```python
from build123d import *

# Parameters (mm, degrees)
CASING_SKETCH_W        = 150
CASING_SKETCH_H        = 200
CASING_DEPTH           = 100
SHELL1_T               = -2
COMPARTMENTS_OUTLINE_W = 146
COMPARTMENTS_OUTLINE_H = 2
COMPARTMENTS_DEPTH     = 100
SKETCH4_W              = 51
SKETCH4_H              = 60
SKETCH4_W_2            = 35
SKETCH4_H_2            = 40
SKETCH4_W_3            = 30
SKETCH4_H_3            = 100
SKETCH4_W_4            = 70
SKETCH4_H_4            = 30
MEDICINES_DEPTH        = 75
SKETCH6_R              = 17.5
SKETCH6_R_2            = 5
BANDAGE_DEPTH          = 75
SKETCH7_R              = 7.5
VIALS_DEPTH            = 25
SKETCH9_W              = 150
SKETCH9_H              = 200
BOSS_EXTRUDE1_DEPTH    = 2
CUT_EXTRUDE1_DEPTH     = 2


# Read off the part's stored shape, not the designer's step: Compartments
with BuildPart() as part:
    # Casing Sketch → Casing (new body)
    with BuildSketch(Plane(origin=(0, 0, 0), x_dir=(1, 0, 0), z_dir=(0, 1, 0))):
        Rectangle(CASING_SKETCH_W, CASING_SKETCH_H)
    extrude(amount=CASING_DEPTH)

    # Shell1
    shell1_openings = [part.faces().sort_by_distance(p)[0] for p in [
        (0, 100, 0),
    ]]
    offset(amount=SHELL1_T, openings=shell1_openings, kind=Kind.INTERSECTION)

    # Compartments outline → Compartments (add)
    with BuildSketch(Plane(origin=(0, 2, 0), x_dir=(1, 0, 0), z_dir=(0, 1, 0))):
        Polygon((-2, 2), (-73, 2), (-73, 0), (0, 0), (0, 98), (-2, 98), align=None)
        with Locations((0, -51)):
            Rectangle(COMPARTMENTS_OUTLINE_W, COMPARTMENTS_OUTLINE_H)
    extrude(amount=COMPARTMENTS_DEPTH)

    # Sketch4 → Medicines (add)
    with BuildSketch(Plane(origin=(0, 2, 0), x_dir=(1, 0, 0), z_dir=(0, 1, 0))):
        with Locations((-37.5, 32)):
            Rectangle(SKETCH4_W, SKETCH4_H)
        with Locations((15.5, -30)):
            Rectangle(SKETCH4_W_2, SKETCH4_H_2)
        with Locations((53, 0)):
            Rectangle(SKETCH4_W_3, SKETCH4_H_3)
        with Locations((-28, -83)):
            Rectangle(SKETCH4_W_4, SKETCH4_H_4)
    extrude(amount=MEDICINES_DEPTH)

    # Sketch6 → Bandage (add)
    with BuildSketch(Plane(origin=(0, 2, 0), x_dir=(1, 0, 0), z_dir=(0, 1, 0))):
        with Locations(Location((43.231606139, -78.51417502, 0), (0, 0, 270))):
            Circle(SKETCH6_R)
        with Locations(Location((43.231606139, -78.51417502, 0), (0, 0, 270))):
            Circle(SKETCH6_R_2, mode=Mode.SUBTRACT)
    extrude(amount=BANDAGE_DEPTH)

    # Sketch7 → Vials (add)
    with BuildSketch(Plane(origin=(0, 0, 50), x_dir=(-1, 0, 0), z_dir=(0, 0, -1))):
        with Locations((61.244974069, 52)):
            Circle(SKETCH7_R)
        with Locations((37.16355204, 52)):
            Circle(SKETCH7_R)
        with Locations((14.684505224, 52)):
            Circle(SKETCH7_R)
    extrude(amount=VIALS_DEPTH)

    # Sketch9 → Boss-Extrude1 (add)
    with BuildSketch(Plane(origin=(0, 100, 0), x_dir=(1, 0, 0), z_dir=(0, 1, 0))):
        Rectangle(SKETCH9_W, SKETCH9_H)
    extrude(amount=BOSS_EXTRUDE1_DEPTH)

    # Sketch10 → Cut-Extrude1 (cut)
    with BuildSketch(Plane(origin=(0, 102, 0), x_dir=(1, 0, 0), z_dir=(0, 1, 0))):
        Polygon((-22.5, 70.520593301), (22.5, 70.520593301), (22.5, 25.520593301), (67.5, 25.520593301), (67.5, -19.479406699), (22.5, -19.479406699), (22.5, -64.479406699), (-22.5, -64.479406699), (-22.5, -19.479406699), (-67.5, -19.479406699), (-67.5, 25.520593301), (-22.5, 25.520593301), align=None)
    extrude(amount=-CUT_EXTRUDE1_DEPTH, mode=Mode.SUBTRACT)


solid = part.part
```
Source: CAD feature listing. Evaluate the final solid. Frame: model axes, mm. A direction names the side the tool comes from. Coordinates: 2 decimals unless noted, no trailing zeros. Loops run counter-clockwise (first coordinate to the right, second up) from the corner with the lowest first, then second, coordinate; pieces in that order, holes last. Notation, with made-up numbers: M -20,-40 L -3,-40 A20 ccw -3,-6 Z; hole C 65,6.5 d6. An arc over 180 degrees is marked long. Use a Markdown table: item, result. Add a question column.
Q1. Draft query along Z for faces 3 (the flat face through (75, 50, 1)), 4 (the flat face through (33, 39, 30)), 5 (the flat face through (-1, 50, 100)). Return one class per face: pulls with the +Z half, pulls with the -Z half, needs draft (parallel to the pull), parting line crosses it, or undercut.
Q2. Material intervals for L1, parallel to Z at x = -23, y = 19; L2, parallel to Z at x = -67, y = 55.5; L3, parallel to Z at x = 12, y = 45, sorted ascending.
Q3. Section query C-C, the plane y = 87. Return loops of the section in (x, z).
Q4. Section query B-B, the plane x = -50. Return loops of the section in (y, z).
Q5. First-contact query: pin 1 (10 mm diameter, centred on x = -3, z = -62.5, fed in from +Y). Flat tip, straight axial feed; report the tip coordinate or a pass-through.
Q6. Section query D-D, the plane z = -81. Return loops of the section in (x, y).
Q7. Section query A-A, the plane z = 35.5. Return loops of the section in (x, y), and give its area (3 significant figures).
Q8. Access query for faces 1 (the flat face through (-1, 100, -20)), 2 (the cylindrical face through (-59.62, 44.68, 37.67)). Directions: +Z, -Z, +X, -X, +Y, -Y. A direction counts if a zero-diameter tool reaches every point of the face in a straight line with its end or side. Return the directions, or none.
Result:
| question | item | result |
|---|---|---|
| 1 | face 3 | needs draft |
| 1 | face 4 | undercut |
| 1 | face 5 | pulls with the +Z half |
| 2 | L1 | z = -100 to -98, -62 to 0, 50 to 52, 68 to 100 |
| 2 | L2 | z = -100 to -98, -2 to 0, 25 to 52, 98 to 100 |
| 2 | L3 | z = -100 to -98, 10 to 52, 98 to 100 |
| 3 | outline | M -75,-100 L 75,-100 L 75,100 L -75,100 Z; hole M -73,-98 L -2,-98 L -2,-2 L -73,-2 Z; hole M -73,0 L 0,0 L 0,-98 L 73,-98 L 73,50 L -73,50 Z; hole M -73,52 L 73,52 L 73,98 L -73,98 Z |
| 4 | outline | M 0,-100 L 102,-100 L 102,-25.52 L 100,-25.52 L 100,-98 L 2,-98 L 2,-62 L 77,-62 L 77,-2 L 100,-2 L 100,0 L 2,0 L 2,50 L 100,50 L 100,19.48 L 102,19.48 L 102,100 L 0,100 Z; hole M 2,52 L 100,52 L 100,98 L 77,98 L 77,68 L 2,68 Z |
| 5 | pin 1 | stops at y = 100 |
| 6 | outline | M -75,0 L 75,0 L 75,102 L -75,102 Z; hole M -73,2 L -2,2 L -2,100 L -73,100 Z; hole M 0,2 L 73,2 L 73,100 L 0,100 Z |
| 7 | outline | M -75,0 L 75,0 L 75,102 L 22.5,102 L 22.5,100 L 73,100 L 73,2 L 68,2 L 68,77 L 38,77 L 38,2 L 33,2 L 33,77 L -2,77 L -2,2 L -73,2 L -73,100 L -22.5,100 L -22.5,102 L -75,102 Z; C -61.24,52 d15; C -37.16,52 d15; C -14.68,52 d15 |
| 7 | area | 6,310 mm2 |
| 8 | face 1 | +Y |
| 8 | face 2 | none |
